Part model, mm, in its own coordinate system. Face numbers are marked on the shaded views. A direction names the side the tool comes from. Coordinates: 2 decimals unless noted, no trailing zeros. Write each loop counter-clockwise with the first axis right and the second up, starting at its lowest first coordinate (ties: lowest second). Pieces come first, ordered by that corner, then holes. Notation, with made-up numbers: M -30.75,16.5 L -9.75,16.5 A9 cw -9.75,23.5 Z; hole C -36.5,20.25 d6. An arc over 180 degrees is marked long. Use a Markdown table: item, result. Add a question column.
Q1. Slice it at B-B on y = 0. Write the cut outline in (x, z), then the cut area to 3 significant figures.
Q2. Wall check: L1, parallel to X at y = 1, z = 3.25; L2, parallel to Y at x = 0, z = 8; L3, parallel to X at y = 0.5, z = 3.5. Give the ranges that are in metal, low to high. Write a range as from..to.
Q3. Slice it at C-C on z = 1. Write the cut outline in (x, y), then the cut area to 3 significant figures.
Q4. Pin check, flat tips, straight feed: pin 1 Ø2 at (x, z) = (1.5, 8) entering from +Y; pin 2 Ø3 at (y, z) = (4, 7) entering from -X; pin 3 Ø5 at (y, z) = (-4, 9.5) entering from +X. Stop position of each tip, or through.
Q5. Tool access for the marked faces 1 and 2: list every direction of +Z, -Z, +X, -X, +Y, -Y with a clear straight run to the whole face (end or side of a thin tool).
Q6. Slice it at A-A on x = 0. Write the cut outline in (y, z), then the cut area to 3 significant figures.
Q7. Slice it at D-D on y = -3.5. Write the cut outline in (x, z), then the cut area to 3 significant figures.
Q8. Mould opens along X. For the marked faces 3, 4 and 5 say: released by +X, released by -X, zero draft, split by the parting line, or undercut.
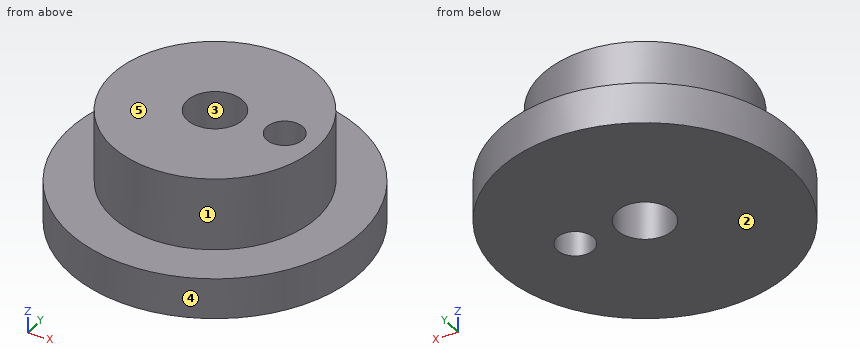
from build123d import *

# Parameters (mm, degrees)
F3_D = 4


with BuildPart() as f1:
    # F0 (on Front) → F1 (revolve)
    with BuildSketch(Plane.XZ):
        Polygon((11.25, 12.5), (3.05, 12.5), (3.05, 0), (16, 0), (16, 4.5), (11.25, 4.5), align=None)
    revolve(axis=Axis((0, 0, 22.5), (0, 0, 1)))

    # F3 (through all)
    with Locations(Plane.XY.offset(12.5)):
        with Locations((7.5, 0)):
            Hole(F3_D / 2)


solid = f1.part
Recorded:
| question | item | result |
|---|---|---|
| 1 | outline | M -16,0 L -3.05,0 L -3.05,12.5 L -11.25,12.5 L -11.25,4.5 L -16,4.5 Z; M 3.05,0 L 5.5,0 L 5.5,12.5 L 3.05,12.5 Z; M 9.5,0 L 16,0 L 16,4.5 L 11.25,4.5 L 11.25,12.5 L 9.5,12.5 Z |
| 1 | area | 198 mm² |
| 2 | L1 | -15.97..-2.88, 2.88..5.77, 9.23..15.97 |
| 2 | L2 | -11.25..-3.05, 3.05..11.25 |
| 2 | L3 | -15.99..-3.01, 3.01..5.56, 9.44..15.99 |
| 3 | outline | C 0,0 d32; hole C 0,0 d6.1; hole C 7.5,0 d4 |
| 3 | area | 762 mm² |
| 4 | pin 1 | y = 11.24 |
| 4 | pin 2 | x = -10.97 |
| 4 | pin 3 | x = 11.15 |
| 5 | face 1 | +Z |
| 5 | face 2 | -Z, +X, -X, +Y, -Y |
| 6 | outline | M -16,0 L -3.05,0 L -3.05,12.5 L -11.25,12.5 L -11.25,4.5 L -16,4.5 Z; M 3.05,0 L 16,0 L 16,4.5 L 11.25,4.5 L 11.25,12.5 L 3.05,12.5 Z |
| 6 | area | 248 mm² |
| 7 | outline | M -15.61,0 L 15.61,0 L 15.61,4.5 L 10.69,4.5 L 10.69,12.5 L -10.69,12.5 L -10.69,4.5 L -15.61,4.5 Z |
| 7 | area | 312 mm² |
| 8 | face 3 | undercut |
| 8 | face 4 | split by the parting line |
| 8 | face 5 | zero draft |
